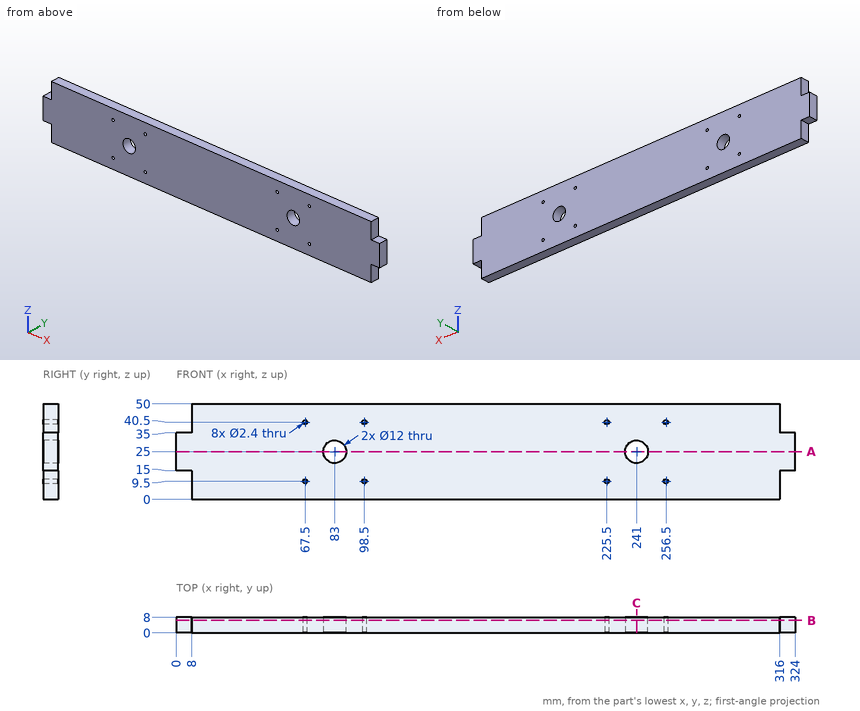
For this review, use the dimensioned drawing (mm, ordinates from the lowest corner) and the shaded views. Give positions to 0.01 mm unless a question says otherwise; leave off trailing zeros. Write each loop counter-clockwise with the first axis right and the second up, starting at its lowest first coordinate (ties: lowest second). Pieces come first, ordered by that corner, then holes.
(1) Consider section C-C, the plane x = 241. Give the boundary of the cut face in (y, z).
(2) Consider section A-A, the plane z = 25. Give the boundary of the cut face in (x, y).
(3) Consider section B-B, the plane y = 6.5. Give the number of separate pieces and of enclosed holes in the cut face, and give its area (3 significant figures).
(4) To check wall thickness, follow L1, parallel to X at y = 5.5, z = 25; L2, parallel to X at y = 4, z = 9.5; L3, parallel to Z at x = 225.5, y = 4. State the ranges of each line that lie inside material, in increasing order.
(5) For P1, Ø4, axis at y = 5.5, z = 12, coming from the +X side; P2, Ø2.5, axis at x = 4, y = 3, coming from the -Z side; P3, Ø2.5, axis at x = 6, y = 3, coming from the +Z side, all flat-tipped, find the tip position at first contact; note any pin that passes through.
Returned:
1. outline: (0, 0) - (8, 0) - (8, 19) - (0, 19) - close; (0, 31) - (8, 31) - (8, 50) - (0, 50) - close
2. outline: (0, 0) - (77, 0) - (77, 8) - (0, 8) - close; (89, 0) - (235, 0) - (235, 8) - (89, 8) - close; (247, 0) - (324, 0) - (324, 8) - (247, 8) - close
3. separate pieces: 1
3. enclosed holes: 10
3. area: 15,500 mm2
4. L1: x = 0 to 77, 89 to 235, 247 to 324
4. L2: x = 8 to 66.3, 68.7 to 97.3, 99.7 to 224.3, 226.7 to 255.3, 257.7 to 316
4. L3: z = 0 to 8.3, 10.7 to 39.3, 41.7 to 50
5. P1: stops at x = 316
5. P2: stops at z = 15
5. P3: stops at z = 35
